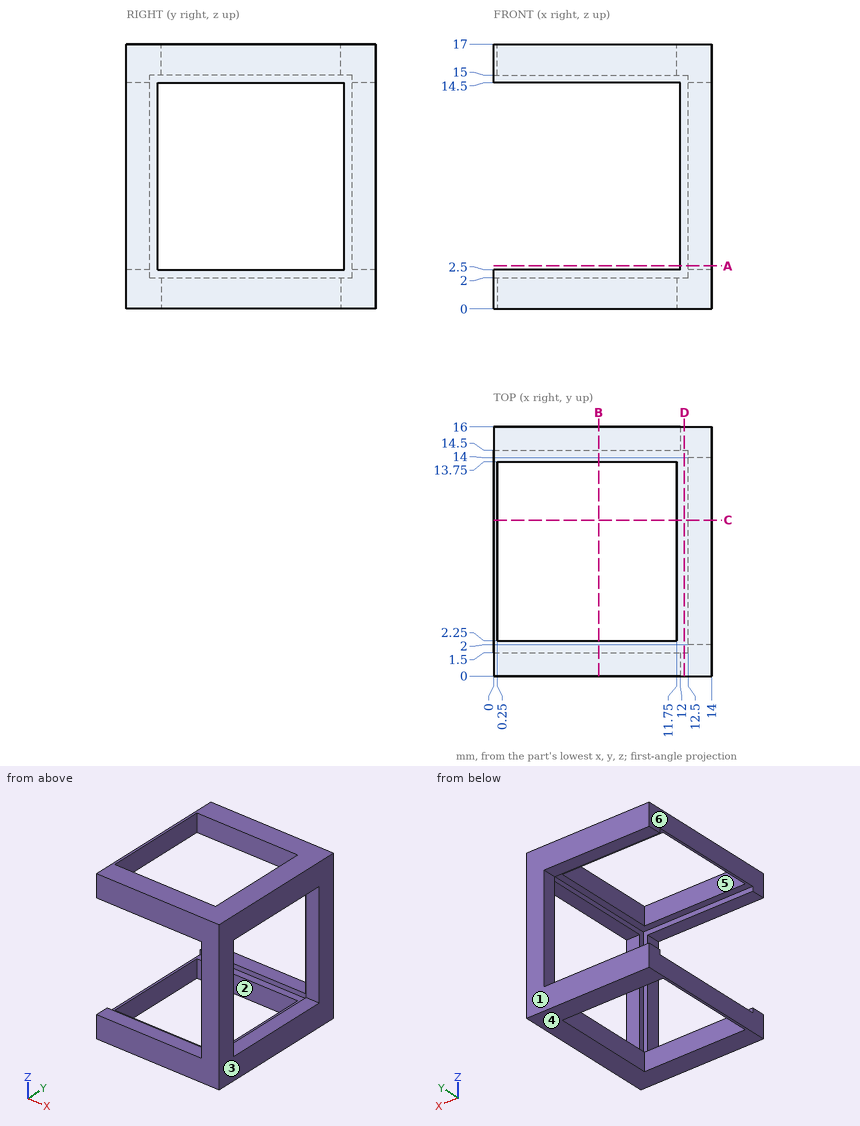
Answer from the drawing. Dimensions are ordinates in mm from the lowest x, y and z of the part. A direction names the side the tool comes from. Coordinates: 2 decimals unless noted, no trailing zeros. Write each loop counter-clockwise with the first axis right and the second up, starting at its lowest first coordinate (ties: lowest second). Pieces come first, ordered by that corner, then holes. Notation, with made-up numbers: (-36.5, 46) - (-29.5, 46) arc R4 ccw to (-29.5, 50) - close; hole circle Ø3 at (87, -26.5). An arc over 180 degrees is marked (long way). Answer as CSV lines item,"result".
1. Straight lines are drawn through the part: line 1 (X direction, y = 12, z = 1.5); line 2 (Y direction, x = 1.5, z = 1); line 3 (X direction, y = 15.25, z = 12). For each, find the intervals that lie inside material, in ascending order. Write a range as [from, to].
Computed values:
line 1,"x = [0, 0.25], [11.75, 14]"
line 2,"y = [0, 2.25], [13.75, 16]"
line 3,"x = [12, 14]"
2. Given P1, Ø1.2, axis at y = 15, z = 7, coming from the -X side; P2, Ø0.6, axis at y = 5.5, z = 0.5, coming from the -X side, each flat-ended and moving along its own axis, determine where each tip first touches the part or whether it passes through.
Computed values:
P1,"stops at x = 12"
P2,"stops at x = 0"
3. Find section C-C (y = 10). Give the vertices of the cut face in (x, z).
Computed values:
outline,"(0, 0) - (0.25, 0) - (0.25, 2) - (0, 2) - close; (0, 15) - (0.25, 15) - (0.25, 17) - (0, 17) - close; (11.75, 0) - (14, 0) - (14, 2.5) - (12.5, 2.5) - (12.5, 2) - (11.75, 2) - close; (11.75, 15) - (12.5, 15) - (12.5, 14.5) - (14, 14.5) - (14, 17) - (11.75, 17) - close"
4. Determine the mould class of the marked faces 3, 4, 5 and 6 for opening direction X: +X half, -X half, draft (parallel to the pull), parting line (faces both ways), or undercut.
Computed values:
face 3,"+X half"
face 4,"draft"
face 5,"undercut"
face 6,"-X half"
5. Find section B-B (x = 6.75). Give the vertices of the cut face in (y, z).
Computed values:
outline,"(0, 0) - (2.25, 0) - (2.25, 2) - (1.5, 2) - (1.5, 2.5) - (0, 2.5) - close; (0, 14.5) - (1.5, 14.5) - (1.5, 15) - (2.25, 15) - (2.25, 17) - (0, 17) - close; (13.75, 0) - (16, 0) - (16, 2.5) - (14.5, 2.5) - (14.5, 2) - (13.75, 2) - close; (13.75, 15) - (14.5, 15) - (14.5, 14.5) - (16, 14.5) - (16, 17) - (13.75, 17) - close"
6. A tool of negligible diameter and unlimited length cuts with its end or side. For the marked faces 1 and 2, from which of +Z, -Z, +X, -X, +Y, -Y can it reach the whole face along a straight path? Write none if from no direction.
Computed values:
face 1,"+Z, -Z, +X, -X, +Y"
face 2,"+Z, -Z"
7. Find section D-D (x = 12.25). Give the vertices of the cut face in (y, z), plus the area to 3 significant figures.
Computed values:
outline,"(0, 0) - (16, 0) - (16, 17) - (0, 17) - close; hole (1.5, 2) - (14.5, 2) - (14.5, 15) - (1.5, 15) - close"
area,"103 mm²"
8. Find section A-A (z = 2.75). Give the vertices of the cut face in (x, y).
Computed values:
outline,"(12, 0) - (14, 0) - (14, 2) - (12.5, 2) - (12.5, 1.5) - (12, 1.5) - close; (12, 14.5) - (12.5, 14.5) - (12.5, 14) - (14, 14) - (14, 16) - (12, 16) - close"
